The drawing under review shows one solid part. Ordinate dimensions are in mm from its lowest x, y, z. Give positions to 0.01 mm unless a question says otherwise; leave off trailing zeros. Loops run counter-clockwise (first coordinate to the right, second up) from the corner with the lowest first, then second, coordinate; pieces in that order, holes last. Notation, with made-up numbers: M -22.75,68.5 L 28.25,68.5 A28 ccw 28.25,91.5 Z; hole C -24.75,20.25 d1. An arc over 180 degrees is marked long. Put each result on its own line as item: value. Start each with the question number.
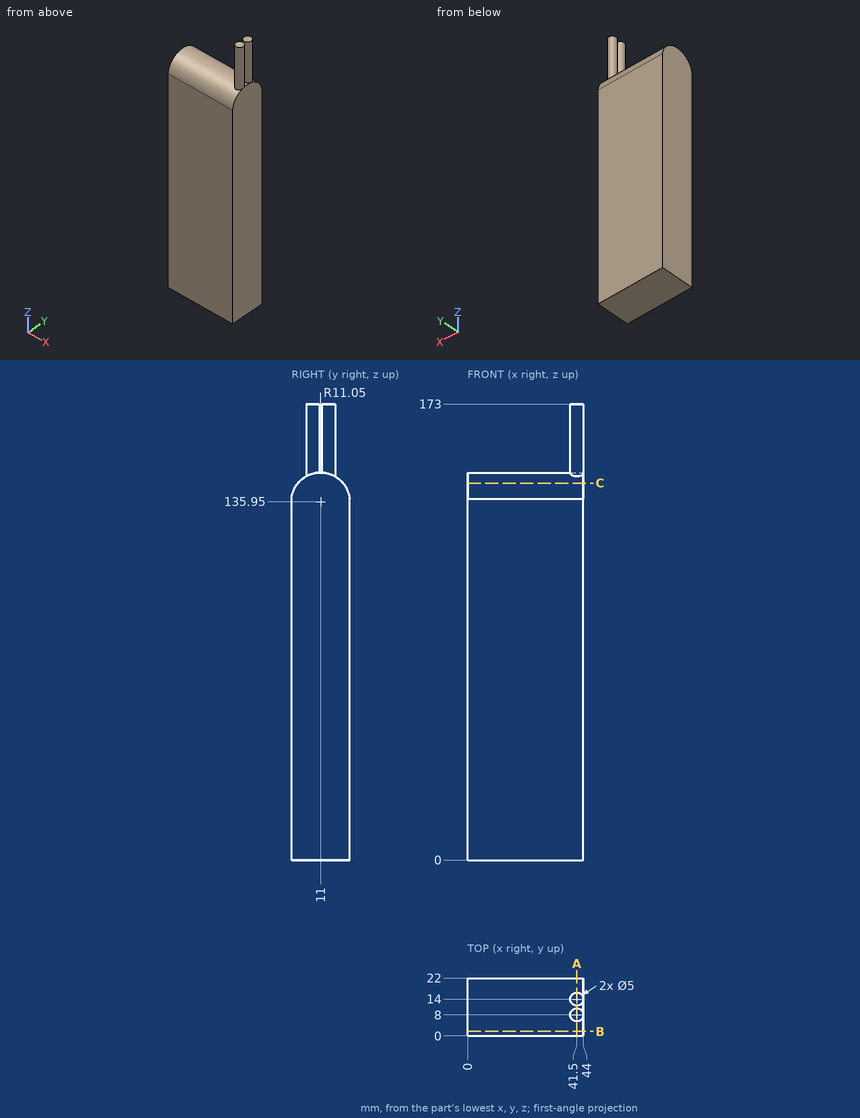
(1) We need section A-A, the plane x = 41.5. Write out the cut boundary in (y, z), plus the area to 3 significant figures.
(2) We need section B-B, the plane y = 1.75. Write out the cut boundary in (x, z), plus the area to 3 significant figures.
(3) To check wall thickness, follow L1, parallel to Z at x = 38.5, y = 10.5; L2, parallel to Z at x = 32.5, y = 16.5. State the ranges of each line that lie inside material, in increasing order. Write a range as [from, to].
(4) We need section C-C, the plane z = 143. Write out the cut boundary in (x, y), plus the area to 3 significant figures.
(5) Insertion check: pin 1 (6 mm diameter, centred on x = 20, y = 8, fed in from +Z); pin 2 (8 mm diameter, centred on x = 39, y = 17.5, fed in from +Z). Each pin has a flat end and moves straight along its axis. Give the tip position at first contact, or say it passes through.
Check sheet entries:
1. outline: M 0,0 L 22,0 L 22,137 A11.05 ccw 16.5,145.53 L 16.5,173 L 11.5,173 L 11.5,146.99 A11.05 ccw 10.5,146.99 L 10.5,173 L 5.5,173 L 5.5,145.53 A11.05 ccw 0,137 Z
1. area: 3,450 mm²
2. outline: M 0,0 L 44,0 L 44,141.99 L 0,141.99 Z
2. area: 6,250 mm²
3. L1: z = [0, 146.99]
3. L2: z = [0, 145.53]
4. outline: M 0,2.49 L 44,2.49 L 44,19.51 L 0,19.51 Z
4. area: 749 mm²
5. pin 1: stops at z = 147
5. pin 2: stops at z = 173
